Work out the finished part from the listing and answer in its coordinate system (mm). A direction names the side the tool comes from. Round coordinates to 2 decimals unless told otherwise and drop trailing zeros. Order: outer loops, then holes, each group sorted by start corner. A loop starts at its lowest first (then second) coordinate and runs counter-clockwise, first axis right, second up. Notation, with made-up numbers: (-12, 74) - (32, 74) arc R4 ccw to (32, 79) - close; hole circle Ø3 at (-12, 28). An arc over 180 degrees is marked (long way). Put each result on its own line as item: value.
```python
from build123d import *

# Parameters (mm, degrees)
F0_W      = 58.42
F0_H      = 19.304
F1_DEPTH  = 104.648
F3_DEPTH  = 254
F4_DEPTH  = 18.796
F2_W      = 10.16
F2_H      = 6.604
F5_DEPTH  = 254
F8_DEPTH  = 25.4
F10_DEPTH = 25.4


with BuildPart() as f1:
    # F0 (on Front) → F1 (new body)
    with BuildSketch(Plane.XZ):
        with Locations((-25.778878, -6.473551)):
            Rectangle(F0_W, F0_H)
    extrude(amount=F1_DEPTH)

    # F2 (on face) → F3 (cut)
    with BuildSketch(Plane.XY.offset(3.178449)):
        with BuildLine():
            ThreePointArc((-35.684878, -76.2), (-25.778878, -86.106), (-15.872878, -76.2))
            Line((-15.872878, -76.2), (-35.684878, -76.2))
        make_face()
        with BuildLine():
            Line((-35.684878, -76.2), (-15.872878, -76.2))
            ThreePointArc((-15.872878, -76.2), (-25.778878, -66.294), (-35.684878, -76.2))
        make_face()
        with BuildLine():
            Line((-35.684878, -104.648), (-25.778878, -104.648))
            Line((-25.778878, -104.648), (-15.872878, -104.648))
            Line((-15.872878, -104.648), (-15.872878, -76.2))
            ThreePointArc((-15.872878, -76.2), (-25.778878, -86.106), (-35.684878, -76.2))
            Line((-35.684878, -76.2), (-35.684878, -104.648))
        make_face()
        Polygon((-54.988878, -104.648), (-47.368878, -104.648), (-54.988878, -56.388), align=None)
        Polygon((3.431122, -56.388), (-4.188878, -104.648), (3.431122, -104.648), align=None)
    extrude(amount=-F3_DEPTH, mode=Mode.SUBTRACT)

    # F2 (on face) → F4 (join)
    with BuildSketch(Plane.XY.offset(3.178449)):
        Polygon((-54.988878, -23.876), (3.431122, -23.876), (3.431122, -6.604), (-6.728878, -6.604), (-6.728878, 0), (-44.828878, 0), (-44.828878, -6.604), (-54.988878, -6.604), align=None)
    extrude(amount=F4_DEPTH)

    # F2 (on face) → F5 (cut)
    with BuildSketch(Plane.XY.offset(3.178449)):
        with BuildLine():
            Line((-35.684878, -104.648), (-25.778878, -104.648))
            Line((-25.778878, -104.648), (-15.872878, -104.648))
            Line((-15.872878, -104.648), (-15.872878, -76.2))
            ThreePointArc((-15.872878, -76.2), (-25.778878, -86.106), (-35.684878, -76.2))
            Line((-35.684878, -76.2), (-35.684878, -104.648))
        make_face()
        with BuildLine():
            Line((-35.684878, -76.2), (-15.872878, -76.2))
            ThreePointArc((-15.872878, -76.2), (-25.778878, -66.294), (-35.684878, -76.2))
        make_face()
        Polygon((-54.988878, -56.388), (-54.988878, -104.648), (-47.368878, -104.648), align=None)
        Polygon((-4.188878, -104.648), (3.431122, -104.648), (3.431122, -56.388), align=None)
        with Locations((-49.908878, -3.302)):
            Rectangle(F2_W, F2_H)
        with Locations((-1.648878, -3.302)):
            Rectangle(F2_W, F2_H)
    extrude(amount=-F5_DEPTH, mode=Mode.SUBTRACT)

    # F7 (on face) → F8 (cut)
    with BuildSketch(Plane(origin=(0, 0, 0), x_dir=(-1, 0, 0), z_dir=(0, 1, 0))):
        Polygon((86.693414, 21.974449), (35.135657, 21.974449), (86.693414, -7.065322), align=None)
    extrude(amount=-F8_DEPTH, mode=Mode.SUBTRACT)

    # F9 (on face) → F10 (cut)
    with BuildSketch(Plane(origin=(0, 0, 0), x_dir=(-1, 0, 0), z_dir=(0, 1, 0))):
        Polygon((-10.884415, 32.844201), (-3.437184, 10.502506), (34.180883, 32.844201), align=None)
    extrude(amount=-F10_DEPTH, mode=Mode.SUBTRACT)


solid = f1.part
```
1) For faces 5 (the flat face through (-26, -55, 3.178)), 6 (the flat face through (-35.685, -90, -6)), 7 (the flat face through (-6.729, -3, 0)), determine the directions among +Z, -Z, +X, -X, +Y, -Y from which every point of the face is accessible in a straight line to the end or side of a thin tool.
Findings below:
face 5: +Z, +X, -X, -Y
face 6: +Z, -Z, -Y
face 7: +Z, -Z, +X, +Y
2) Straight lines are drawn through the part: L1, parallel to Y at x = -46.5, z = 15.5; L2, parallel to Y at x = -13.5, z = 19.5; L3, parallel to X at y = -87, z = -9. For each, find the intervals that lie inside material, in ascending order. Write a range as from..to.
Findings below:
L1: y = -23.88..-6.6
L2: y = -23.88..0
L3: x = -50.16..-35.68, -15.87..-1.4
3) Given pin 1 Ø15.5 at (y, z) = (-96.5, -2.5) entering from +X; pin 2 Ø4 at (x, y) = (-34, -72.5) entering from +Z; pin 3 Ø5 at (x, z) = (0, 1.5) entering from +Y, each flat-ended and moving along its own axis, determine where each tip first touches the part or whether it passes through.
Findings below:
pin 1: stops at x = -1.68
pin 2: stops at z = 3.18
pin 3: stops at y = -6.6
4) For a pull along X with two mould halves and no side action, classify faces 1 (the flat face through (-2, -6.604, 0)), 2 (the flat face through (-54.989, -31, -6)), 3 (the flat face through (-15.873, -91, -6)), 4 (the cylindrical face through (-25.561, -66.296, -6.338)) as pulls with the +X half, pulls with the -X half, needs draft (parallel to the pull), parting line crosses it, or undercut.
Findings below:
face 1: needs draft
face 2: pulls with the -X half
face 3: undercut
face 4: undercut
5) A cutting plane is placed at D-D on y = -50.5. Write down the section's boundary in (x, z), then the cut area to 3 significant figures.
Findings below:
outline: (-54.99, -16.13) - (3.43, -16.13) - (3.43, 3.18) - (-54.99, 3.18) - close
area: 1,130 mm2
6) A cutting plane is placed at C-C on x = -11. Write down the section's boundary in (y, z).
Findings below:
outline: (-104.65, -16.13) - (0, -16.13) - (0, 19.08) - (-23.88, 19.08) - (-23.88, 3.18) - (-104.65, 3.18) - close
7) A cutting plane is placed at A-A on y = -75. Write down the section's boundary in (x, z).
Findings below:
outline: (-52.05, -16.13) - (-35.61, -16.13) - (-35.61, 3.18) - (-52.05, 3.18) - close; (-15.95, -16.13) - (0.49, -16.13) - (0.49, 3.18) - (-15.95, 3.18) - close
8) A cutting plane is placed at B-B on z = 1. Write down the section's boundary in (x, y).
Findings below:
outline: (-54.99, -56.39) - (-47.37, -104.65) - (-35.68, -104.65) - (-35.68, -76.2) arc R9.91 cw to (-15.87, -76.2) - (-15.87, -104.65) - (-4.19, -104.65) - (3.43, -56.39) - (3.43, -6.6) - (-6.73, -6.6) - (-6.73, 0) - (-44.83, 0) - (-44.83, -6.6) - (-54.99, -6.6) - close
